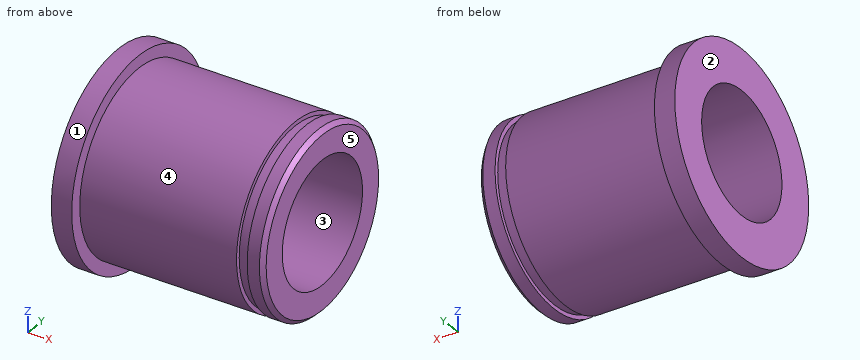
```python
from build123d import *

# Parameters (mm, degrees)
F2_SIZE = 0.5
F3_W    = 1.3
F3_H    = 0.5


with BuildPart() as f1:
    # F0 (on Top) → F1 (revolve)
    with BuildSketch(Plane.XY):
        Polygon((0, 12.5), (0, 7.5), (25, 7.5), (25, 11), (2.5, 11), (2.5, 12.5), align=None)
    revolve(axis=Axis((6.446342, 0, 0), (1, 0, 0)))

    # F2
    f2_edges = [f1.edges().sort_by_distance(p)[0] for p in [
        (25, -11, 0),
    ]]
    chamfer(f2_edges, length=F2_SIZE)

    # F3 (on Front) → F4 (revolve, cut)
    with BuildSketch(Plane.XZ):
        with Locations((22.35, 10.75)):
            Rectangle(F3_W, F3_H)
    revolve(axis=Axis((15.843794, 0, 0), (1, 0, 0)), mode=Mode.SUBTRACT)


solid = f1.part
```
Build history of the part. All positions in model axes, mm. Face numbers are marked on the shaded views. A direction names the side the tool comes from. Round coordinates to 2 decimals unless told otherwise and drop trailing zeros. Order: outer loops, then holes, each group sorted by start corner. A loop starts at its lowest first (then second) coordinate and runs counter-clockwise, first axis right, second up. Notation, with made-up numbers: (63.25, 37.25) -> (82.25, 37.25) arc R29 cw to (82.25, 68.25) -> close; hole circle Ø5 at (38.25, 25.25). An arc over 180 degrees is marked (long way). Answer in a Markdown table with one row per item.
1) Band-saw the part on C-C on x = 10.75. Give the cut face in (y, z).
Values:
| item | result |
|---|---|
| outline | circle Ø22 at (0, 0); hole circle Ø15 at (0, 0) |
2) Band-saw the part on D-D on x = 22.25. Give the cut face in (y, z).
Values:
| item | result |
|---|---|
| outline | circle Ø21 at (0, 0); hole circle Ø15 at (0, 0) |
3) Pin check, flat tips, straight feed: P1, Ø5, axis at x = 8, z = 0, coming from the +Y side; P2, Ø4, axis at x = 19, z = 2, coming from the -Y side; P3, Ø4, axis at x = 16, y = -6, coming from the +Z side. Stop position of each tip, or through.
Values:
| item | result |
|---|---|
| P1 | y = 11 |
| P2 | y = -11 |
| P3 | z = 10.25 |
4) Mould opens along Z. For the marked faces 1, 2 and 3 say: released by +Z, released by -Z, zero draft, split by the parting line, or undercut.
Values:
| item | result |
|---|---|
| face 1 | split by the parting line |
| face 2 | zero draft |
| face 3 | undercut |
5) Wall check: L1, parallel to Z at x = 18, y = 0; L2, parallel to X at y = 10.25, z = 6. Give the ranges that are in metal, low to high.
Values:
| item | result |
|---|---|
| L1 | -11 to -7.5, 7.5 to 11 |
| L2 | 0 to 2.5 |
6) Which spindle directions (+Z, -Z, +X, -X, +Y, -Y) get a long thin tool onto all of the face, cutting with end or side? Do the marked faces 4 and 5. Say none if no direction does.
Values:
| item | result |
|---|---|
| face 4 | +X |
| face 5 | +Z, -Z, +X, +Y, -Y |
7) Band-saw the part on A-A on y = 0. Give the cut face in (x, z), and give its area (3 significant figures).
Values:
| item | result |
|---|---|
| outline | (0, -12.5) -> (2.5, -12.5) -> (2.5, -11) -> (21.7, -11) -> (21.7, -10.5) -> (23, -10.5) -> (23, -11) -> (24.5, -11) -> (25, -10.5) -> (25, -7.5) -> (0, -7.5) -> close; (0, 7.5) -> (25, 7.5) -> (25, 10.5) -> (24.5, 11) -> (23, 11) -> (23, 10.5) -> (21.7, 10.5) -> (21.7, 11) -> (2.5, 11) -> (2.5, 12.5) -> (0, 12.5) -> close |
| area | 181 mm2 |
